Autodesk Inventor part; units mm, degrees
ref_plane "YZ Plane" through (0, 0, 0) normal (1, 0, 0) x (0, 1, 0)
ref_plane "XZ Plane" through (0, 0, 0) normal (0, 1, 0) x (-1, 0, 0)
ref_plane "XY Plane" through (0, 0, 0) normal (0, 0, 1) x (1, 0, 0)
ref_plane "Work Plane1" through (0, 0, 0) normal (0, 0, 1) x (1, 0, 0)
sketch "Sketch1" plane through (0, 0, 0) normal (0, 0, 1) x (1, 0, 0)
  line L0 (0, 2) -> (80.5, 2)
  line L1 (0, -8) -> (0, 2)
  line L2 (82.5, 2) -> (82.5, -98)
  line L3 (82.5, -98) -> (72.5, -98)
  circle A0 centre (76.5, -93) radius 0.75
  circle A1 centre (76.5, -48) radius 0.75
  circle A2 centre (70.5, -4) radius 0.75
  circle A3 centre (40.25, -4) radius 0.75
  circle A4 centre (5, -4) radius 0.75
  line L4 (0, 2) -> (82.5, 2)
  line L5 (82.5, 2) -> (82.5, -98)
  line L6 (82.5, -98) -> (0, -98)
  line L7 (0, -98) -> (0, 2)
  point P0 (0, 0)
extrude "Extrusion1" add sketch "Sketch1" along normal blind 2
sketch "Sketch2" plane through (0, 0, 2) normal (0, 0, 1) x (1, 0, 0)
  circle A0 centre (76.5, -93) radius 0.75
  circle A1 centre (76.5, -93) radius 1.25
  circle A2 centre (76.5, -48) radius 0.75
  circle A3 centre (76.5, -48) radius 1.25
  circle A4 centre (70.5, -4) radius 0.75
  circle A5 centre (70.5, -4) radius 1.25
  circle A6 centre (40.25, -4) radius 0.75
  circle A7 centre (40.25, -4) radius 1.25
  circle A8 centre (5, -4) radius 0.75
  circle A9 centre (5, -4) radius 1.25
  point P0 (0, 0)
  dimension "d2" = 2.5
  dimension "d3" = 2.5
  dimension "d4" = 2.5
  dimension "d5" = 2.5
  dimension "d6" = 2.5
extrude "Extrusion2" cut sketch "Sketch2" against normal blind 2
sketch "Sketch3" plane through (0, -98, 0) normal (-1, 0, 0) x (0, 0, 1)
  line L0 (0, 45) -> (-5, 45)
  line L1 (0, 55) -> (-5, 55)
  line L2 (0, 45) -> (-8, 45)
  line L3 (-8, 45) -> (-8, 55)
  line L4 (-8, 55) -> (0, 55)
  line L5 (0, 55) -> (0, 45)
  circle A0 centre (-4, 50) radius 0.75
  point P0 (0, 98)
  dimension "d9" = 8
  dimension "d10" = 10
  dimension "d11" = 8
  dimension "d13" = 1.5
extrude "Extrusion3" add sketch "Sketch3" against normal blind 5
sketch "Sketch4" plane through (0, -98, 2) normal (-1, 0, 0) x (0, 0, 1)
  line L0 (-2, 0) -> (0, 0)
  line L1 (-2, 0) -> (-10, 0)
  line L2 (-10, 0) -> (-10, 10)
  line L3 (-10, 10) -> (-2, 10)
  line L4 (-2, 10) -> (-2, 0)
  circle A0 centre (-6, 5) radius 0.75
  point P0 (-2, 98)
  dimension "d16" = 8
  dimension "d17" = 10
  dimension "d19" = 1.5
extrude "Extrusion4" add sketch "Sketch4" against normal blind 5
sketch "Sketch5" plane through (0, -98, 2) normal (0, -1, 0) x (1, 0, 0)
  line L0 (82.5, -2) -> (5, -2)
  line L1 (5, -2) -> (15, -2)
  line L2 (15, -2) -> (15, -10)
  line L3 (15, -10) -> (5, -10)
  line L4 (5, -10) -> (5, -2)
  circle A0 centre (10, -6) radius 0.75
  line L5 (45.25, -2) -> (45.25, -7)
  line L6 (35.25, -2) -> (35.25, -7)
  line L7 (35.25, -2) -> (45.25, -2)
  line L8 (45.25, -2) -> (45.25, -10)
  line L9 (45.25, -10) -> (35.25, -10)
  line L10 (35.25, -10) -> (35.25, -2)
  circle A1 centre (40.25, -6) radius 0.75
  point P0 (0, -2)
  dimension "d22" = 10
  dimension "d23" = 8
  dimension "d25" = 1.5
  dimension "d27" = 1.5
extrude "Extrusion5" add sketch "Sketch5" against normal blind 5
sketch "Sketch6" plane through (0, 0, 2) normal (0, 0, 1) x (1, 0, 0)
  point P0 (0, 0)
sketch "Sketch7" plane through (0, 0, 2) normal (0, 0, 1) x (1, 0, 0)
  point P0 (0, 0)
sketch "Sketch8" plane through (0, -53, -8) normal (0, 0, -1) x (-1, 0, 0)
  line L0 (-5, 10) -> (0, 10)
  line L1 (0, 0) -> (0, 10)
  line L2 (-5, 10) -> (0, 10)
  line L3 (0, 10) -> (0, 0)
  line L4 (0, 0) -> (-5, 0)
  line L5 (-5, 0) -> (-5, 10)
  point P0 (0, 53)
extrude "Extrusion6" cut sketch "Sketch8" against normal blind 8
sketch "Sketch9" plane through (0, 0, 0) normal (0, 0, -1) x (-1, 0, 0)
  circle A0 centre (-76.5, -48) radius 1.25
  line L0 (0, 2) -> (0, -98)
  line L1 (0, -53) -> (0, -63)
  line L2 (0, -63) -> (-8, -63)
  line L3 (-8, -63) -> (-8, -53)
  line L4 (-8, -53) -> (0, -53)
  point P0 (0, 0)
  dimension "d33" = 10
  dimension "d34" = 8
  dimension "d35" = 10
extrude "Extrusion7" add sketch "Sketch9" along normal blind 8 contours L0 L2 L3 L4
sketch "Sketch10" plane through (0, 0, -8) normal (0, 0, -1) x (-1, 0, 0)
  line L0 (0, -88) -> (0, -63)
  line L1 (-8, -53) -> (0, -53)
  line L2 (0, -53) -> (0, -63)
  line L3 (0, -63) -> (-8, -63)
  line L4 (-8, -63) -> (-8, -53)
  point P0 (0, 0)
extrude "Extrusion8" cut sketch "Sketch10" against normal blind 8
sketch "Sketch11" plane through (0, 0, 0) normal (0, 0, -1) x (-1, 0, 0)
  circle A0 centre (-76.5, -48) radius 1.25
  line L0 (0, -48) -> (0, -33)
  line L1 (0, 2) -> (0, -98)
  line L2 (0, -33) -> (-8, -33)
  line L3 (-8, -33) -> (-8, -43)
  line L4 (-8, -43) -> (0, -43)
  point P0 (0, 0)
  dimension "d42" = 15
  dimension "d43" = 8
  dimension "d44" = 10
extrude "Extrusion9" add sketch "Sketch11" along normal blind 8 contours L4 L3 L2 L0
sketch "Sketch12" plane through (0, 0, -8) normal (0, 0, -1) x (-1, 0, 0)
  point P0 (0, 0)
sketch "Sketch13" plane through (0, -98, 2) normal (-1, 0, 0) x (0, 0, 1)
  point P0 (-2, 98)
sketch "Sketch14" plane through (0, -98, 2) normal (-1, 0, 0) x (0, 0, 1)
  line L0 (-10, 65) -> (-10, 55)
  circle A0 centre (-6, 60) radius 0.75
  point P0 (-2, 98)
  dimension "d50" = 1.5
extrude "Extrusion10" cut sketch "Sketch14" against normal blind 8
properties part number "Lado izquierdo" material "Nylon 6/6"
Work out the finished part from the listing and answer in its coordinate system (mm). A direction names the side the tool comes from. Give positions to 0.01 mm unless a question says otherwise; leave off trailing zeros. Write each loop counter-clockwise with the first axis right and the second up, starting at its lowest first coordinate (ties: lowest second). Pieces come first, ordered by that corner, then holes. Notation, with made-up numbers: (65, 20.25) -> (110, 20.25) arc R23 cw to (110, 58.25) -> close; hole circle Ø9 at (-31.75, 63.5). An arc over 180 degrees is marked (long way). Write item = value, one per line.
Q1. Section A-A on x = 76.5 is taken. Determine the outline of the cut face in (y, z), and give its area (3 significant figures).
Computed values:
outline = (-98, 0) -> (-94.25, 0) -> (-94.25, 2) -> (-98, 2) -> close; (-91.75, 0) -> (-49.25, 0) -> (-49.25, 2) -> (-91.75, 2) -> close; (-46.75, 0) -> (2, 0) -> (2, 2) -> (-46.75, 2) -> close
area = 190 mm^2
Q2. Section C-C on z = -6.5 is taken. Determine the outline of the cut face in (x, y).
Computed values:
outline = (0, -98) -> (15, -98) -> (15, -93) -> (5, -93) -> (5, -88) -> (0, -88) -> close; (0, -43) -> (8, -43) -> (8, -33) -> (0, -33) -> close; (35.25, -98) -> (45.25, -98) -> (45.25, -93) -> (35.25, -93) -> close
Q3. For a pull along X with two mould halves and no side action, classify faces 5 (the flat face through (0, -58.4, 0.3)), 6 (the cylindrical face through (77.69, -47.62, 1.01)), 7 (the flat face through (4, -33, -4)) as pulls with the +X half, pulls with the -X half, needs draft (parallel to the pull), parting line crosses it, or undercut.
Computed values:
face_5 = pulls with the -X half
face_6 = undercut
face_7 = needs draft
Q4. Section D-D on y = -4 is taken. Determine the outline of the cut face in (x, z).
Computed values:
outline = (0, 0) -> (3.75, 0) -> (3.75, 2) -> (0, 2) -> close; (6.25, 0) -> (39, 0) -> (39, 2) -> (6.25, 2) -> close; (41.5, 0) -> (69.25, 0) -> (69.25, 2) -> (41.5, 2) -> close; (71.75, 0) -> (82.5, 0) -> (82.5, 2) -> (71.75, 2) -> close
Q5. Section B-B on y = -48 is taken. Determine the outline of the cut face in (x, z), and give its area (3 significant figures).
Computed values:
outline = (0, 0) -> (75.25, 0) -> (75.25, 2) -> (0, 2) -> close; (77.75, 0) -> (82.5, 0) -> (82.5, 2) -> (77.75, 2) -> close
area = 160 mm^2
Q6. A tool of negligible diameter and unlimited length cuts with its end or side. For faces 1 (the flat face through (15, -96, -4)), 2 (the flat face through (40, -93, -3)), 3 (the flat face through (2, -88, -4)), 4 (the flat face through (45.25, -96, -4)), from which of +Z, -Z, +X, -X, +Y, -Y can it reach the whole face along a straight path? Write none if from no direction.
Computed values:
face_1 = -Z, +Y, -Y
face_2 = -Z, +X, +Y
face_3 = -Z, +X, -X
face_4 = -Z, +X, +Y, -Y
Q7. Consider line 1 along Y through (x, z) = (3, -4); line 2 along X through (y, z) = (-93, 1.4); line 3 along Z through (x, y) = (5, -38). Determine where each line is inside the solid, lowest interval first.
Computed values:
line_1 = -98 to -93.75, -92.25 to -88, -43 to -38.75, -37.25 to -33
line_2 = 0 to 75.25, 77.75 to 82.5
line_3 = -8 to -4.75, -3.25 to 2
Q8. Flat-ended cylindrical pins translate along their axes: pin 1 Ø4 at (x, z) = (3, -2.5) entering from +Y; pin 2 Ø2 at (x, y) = (76.5, -48) entering from -Z; pin 3 Ø1.5 at (y, z) = (-96.5, -4) entering from +X. Find the tip coordinate at first contact, or state that the pin passes through.
Computed values:
pin_1 = -33
pin_2 = through
pin_3 = 45.25
